```python
from build123d import *

# Parameters (mm, degrees)
EXTRUDE_2_DEPTH = 15
EXTRUDE_3_DEPTH = 2
EXTRUDE_4_DEPTH = 22


with BuildPart() as part:
    # 草图1 → 凸台-拉伸2 (new body)
    with BuildSketch(Plane(origin=(0, 0, 0), x_dir=(1, 0, 0), z_dir=(0, 1, 0))):
        with BuildLine():
            Line((-4.329004892, 2.501942574), (-4.329004892, -2.501942574))
            ThreePointArc((-4.329004892, -2.501942574), (5, 0), (-4.329004892, 2.501942574))
        make_face()
        with BuildLine():
            Line((-1.472222222, 2.203420461), (-1.472222222, -2.203420461))
            ThreePointArc((-1.472222222, -2.203420461), (2.65, 0), (-1.472222222, 2.203420461))
        make_face(mode=Mode.SUBTRACT)
    extrude(amount=EXTRUDE_2_DEPTH)

    # 草图2 → 凸台-拉伸3 (add)
    with BuildSketch(Plane(origin=(0, 15, 0), x_dir=(1, 0, 0), z_dir=(0, 1, 0))):
        with BuildLine():
            Line((-4.329004892, 2.501942574), (-4.329004892, -2.501942574))
            ThreePointArc((-4.329004892, -2.501942574), (5, 0), (-4.329004892, 2.501942574))
        make_face()
    extrude(amount=EXTRUDE_3_DEPTH)

    # 草图3 → 凸台-拉伸4 (add)
    with BuildSketch(Plane(origin=(0, 17, 0), x_dir=(1, 0, 0), z_dir=(0, 1, 0))):
        Polygon((-7.5, 0), (-7.5, 1.8), (-1.8, 1.8), (-1.8, 7.5), (0, 7.5), (1.8, 7.5), (1.8, 1.8), (7.5, 1.8), (7.5, -1.8), (1.8, -1.8), (1.8, -7.5), (-1.8, -7.5), (-1.8, -1.8), (-7.5, -1.8), align=None)
    extrude(amount=EXTRUDE_4_DEPTH)


solid = part.part
```
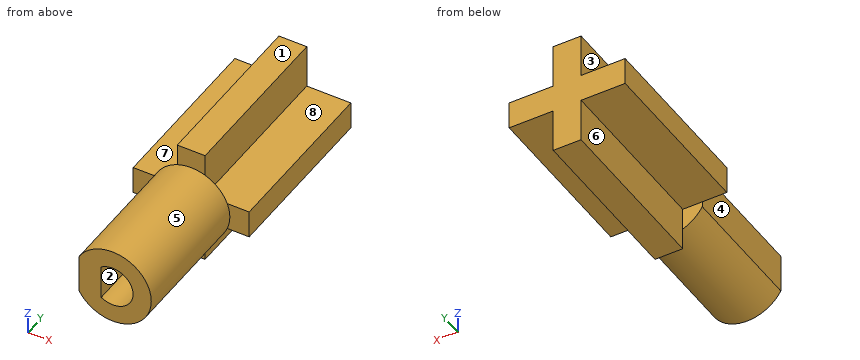
Geometry check sheet. Reference: the model listing, model coordinates, mm. Face numbers are marked on the shaded views. A direction names the side the tool comes from. Round coordinates to 2 decimals unless told otherwise and drop trailing zeros. Write each loop counter-clockwise with the first axis right and the second up, starting at its lowest first coordinate (ties: lowest second). Pieces come first, ordered by that corner, then holes. Notation, with made-up numbers: (57.5, 84) -> (97.5, 84) arc R10 ccw to (97.5, 98) -> close; hole circle Ø11 at (13, 15). An arc over 180 degrees is marked (long way). Put each result on its own line as item: value.
1) Depth check by flat-ended pin: P1, Ø3, axis at x = -4, y = 27.5, coming from the -Z side; P2, Ø4, axis at y = 34.5, z = -5.5, coming from the +X side; P3, Ø4.5, axis at y = 26.5, z = -5.5, coming from the -X side. Enter the tip coordinate at first touch or a pass-through.
Recorded:
P1: stops at z = -1.8
P2: stops at x = 1.8
P3: stops at x = -1.8
2) Cross-section at A-A, the plane x = 0. Enter the section's corners in (y, z), plus the area to 4 significant figures.
Recorded:
outline: (0, -5) -> (17, -5) -> (17, -7.5) -> (39, -7.5) -> (39, 7.5) -> (17, 7.5) -> (17, 5) -> (0, 5) -> (0, 2.65) -> (15, 2.65) -> (15, -2.65) -> (0, -2.65) -> close
area: 420.5 mm2
3) Cross-section at D-D, the plane z = -3.5. Enter the section's corners in (x, y).
Recorded:
outline: (-3.57, 0) -> (3.57, 0) -> (3.57, 17) -> (1.8, 17) -> (1.8, 39) -> (-1.8, 39) -> (-1.8, 17) -> (-3.57, 17) -> close
4) Cross-section at C-C, the plane y = 13.5. Enter the section's corners in (x, z), plus the area to 3 significant figures.
Recorded:
outline: (-4.33, -2.5) arc R5 ccw (long way) to (-4.33, 2.5) -> close; hole (-1.47, -2.2) arc R2.65 ccw (long way) to (-1.47, 2.2) -> close
area: 57.9 mm2
5) Release check for a two-part mould opening along Z. For the marked faces 1, 2 and 3 record: pulls with the +Z half, pulls with the -Z half, needs draft (parallel to the pull), parting line crosses it, or undercut.
Recorded:
face 1: pulls with the +Z half
face 2: undercut
face 3: needs draft
6) Access from +Z, -Z, +X, -X, +Y, -Y to the whole of each face (thin tool, end or side, straight path). Record for the marked faces 4, 5, 6, 7 and 8.
Recorded:
face 4: +Z, -Z, -X, -Y
face 5: -Y
face 6: -Z, -X, +Y
face 7: +Z, -X, +Y
face 8: +Z, +X, +Y
7) Cross-section at B-B, the plane y = 23. Enter the section's corners in (x, z).
Recorded:
outline: (-7.5, -1.8) -> (-1.8, -1.8) -> (-1.8, -7.5) -> (1.8, -7.5) -> (1.8, -1.8) -> (7.5, -1.8) -> (7.5, 1.8) -> (1.8, 1.8) -> (1.8, 7.5) -> (-1.8, 7.5) -> (-1.8, 1.8) -> (-7.5, 1.8) -> close
8) Thickness scan on probe 1 along X at (y, z) = (11.75, 0); probe 2 along Z at (x, y) = (0, 8.5); probe 3 along Y at (x, z) = (-1, -1.5). Record the ranges inside material, lowest first. Write a range as from..to.
Recorded:
probe 1: x = -4.33..-1.47, 2.65..5
probe 2: z = -5..-2.65, 2.65..5
probe 3: y = 15..39
